Verification items for the finished model (mm, model axes). Face numbers are marked on the shaded views. A direction names the side the tool comes from. Coordinates: 2 decimals unless noted, no trailing zeros. Write each loop counter-clockwise with the first axis right and the second up, starting at its lowest first coordinate (ties: lowest second). Pieces come first, ordered by that corner, then holes.
```python
from build123d import *

# Parameters (mm, degrees)
SKETCH_1_W           = 36
SKETCH_1_H           = 20
EXTRUDE_1_DEPTH      = 8
SKETCH_2_W           = 8
SKETCH_2_H           = 20
CUT_EXTRUDE_1_DEPTH  = 3.5
SKETCH_3_R           = 2.5
CUT_EXTRUDE_2_DEPTH  = 4
SKETCH_5_W           = 7
SKETCH_5_H           = 16
CUT_EXTRUDE_4_DEPTH  = 3.5
FILLET_1_R           = 1
SKETCH_6_R           = 1.15
CUT_EXTRUDE_5_DEPTH  = 5.5
SKETCH_7_W           = 10
SKETCH_7_H           = 20
CUT_EXTRUDE_6_DEPTH  = 2
CUT_EXTRUDE_7_DEPTH  = 4
SKETCH_9_R           = 1
CUT_EXTRUDE_10_DEPTH = 3
SKETCH_10_R          = 2
CUT_EXTRUDE_11_DEPTH = 2.4
SKETCH_11_W          = 6
SKETCH_11_H          = 6
CUT_EXTRUDE_15_DEPTH = 3


with BuildPart() as part:
    # 草图1 → 凸台-拉伸1 (new body)
    with BuildSketch(Plane(origin=(0, 0, 0), x_dir=(1, 0, 0), z_dir=(0, 1, 0))):
        with Locations((-18, 10)):
            Rectangle(SKETCH_1_W, SKETCH_1_H)
    extrude(amount=EXTRUDE_1_DEPTH)

    # 草图2 → 切除-拉伸1 (cut)
    with BuildSketch(Plane(origin=(0, 8, 0), x_dir=(1, 0, 0), z_dir=(0, 1, 0))):
        with Locations((-18, 10)):
            Rectangle(SKETCH_2_W, SKETCH_2_H)
    extrude(amount=-CUT_EXTRUDE_1_DEPTH, mode=Mode.SUBTRACT)

    # 草图3 → 切除-拉伸2 (cut)
    with BuildSketch(Plane(origin=(0, 0, 0), x_dir=(-1, 0, 0), z_dir=(0, -1, 0))):
        with Locations((8, 10)):
            Circle(SKETCH_3_R)
        with Locations((28, 10)):
            Circle(SKETCH_3_R)
    extrude(amount=-CUT_EXTRUDE_2_DEPTH, mode=Mode.SUBTRACT)

    # 草图5 → 切除-拉伸4 (cut)
    with BuildSketch(Plane(origin=(0, 8, 0), x_dir=(1, 0, 0), z_dir=(0, 1, 0))):
        with Locations((-25.5, 10)):
            Rectangle(SKETCH_5_W, SKETCH_5_H)
    extrude(amount=-CUT_EXTRUDE_4_DEPTH, mode=Mode.SUBTRACT)

    # 圆角1
    fillet_1_edges = [part.edges().sort_by_distance(p)[0] for p in [
        (-29, 6.25, -2),
        (-29, 6.25, -18),
    ]]
    fillet(fillet_1_edges, radius=FILLET_1_R)

    # 草图6 → 切除-拉伸5 (cut, through all)
    with BuildSketch(Plane(origin=(0, 4.5, 0), x_dir=(1, 0, 0), z_dir=(0, 1, 0))):
        with Locations((-18, 12.5)):
            Circle(SKETCH_6_R)
        with Locations((-18, 7.5)):
            Circle(SKETCH_6_R)
    extrude(amount=-CUT_EXTRUDE_5_DEPTH, mode=Mode.SUBTRACT)

    # 草图7 → 切除-拉伸6 (cut)
    with BuildSketch(Plane(origin=(0, 8, 0), x_dir=(1, 0, 0), z_dir=(0, 1, 0))):
        with Locations((-5, 10)):
            Rectangle(SKETCH_7_W, SKETCH_7_H)
    extrude(amount=-CUT_EXTRUDE_6_DEPTH, mode=Mode.SUBTRACT)

    # 草图8 → 切除-拉伸7 (cut)
    with BuildSketch(Plane(origin=(0, 8, 0), x_dir=(1, 0, 0), z_dir=(0, 1, 0))):
        with BuildLine():
            Line((-24, 18), (-10, 18))
            ThreePointArc((-10, 18), (-9.5, 17.5), (-10, 17))
            Line((-10, 17), (-24, 17))
            ThreePointArc((-24, 17), (-24.5, 17.5), (-24, 18))
        make_face()
    extrude(amount=-CUT_EXTRUDE_7_DEPTH, mode=Mode.SUBTRACT)

    # 草图9 → 切除-拉伸10 (cut)
    with BuildSketch(Plane(origin=(0, 6, 0), x_dir=(1, 0, 0), z_dir=(0, 1, 0))):
        with Locations((-2.25, 2)):
            Circle(SKETCH_9_R)
        with Locations((-7.75, 2)):
            Circle(SKETCH_9_R)
        with Locations((-2.25, 14)):
            Circle(SKETCH_9_R)
        with Locations((-7.75, 14)):
            Circle(SKETCH_9_R)
    extrude(amount=-CUT_EXTRUDE_10_DEPTH, mode=Mode.SUBTRACT)

    # 草图10 → 切除-拉伸11 (cut)
    with BuildSketch(Plane(origin=(0, 0, 0), x_dir=(-1, 0, 0), z_dir=(0, -1, 0))):
        with Locations((18, 12.5)):
            Circle(SKETCH_10_R)
        with Locations((18, 7.5)):
            Circle(SKETCH_10_R)
    extrude(amount=-CUT_EXTRUDE_11_DEPTH, mode=Mode.SUBTRACT)

    # 草图11 → 切除-拉伸15 (cut)
    with BuildSketch(Plane(origin=(0, 0, -20), x_dir=(-1, 0, 0), z_dir=(0, 0, -1))):
        with Locations((3, 3)):
            Rectangle(SKETCH_11_W, SKETCH_11_H)
        with Locations((33, 3)):
            Rectangle(SKETCH_11_W, SKETCH_11_H)
    extrude(amount=-CUT_EXTRUDE_15_DEPTH, mode=Mode.SUBTRACT)


solid = part.part
```
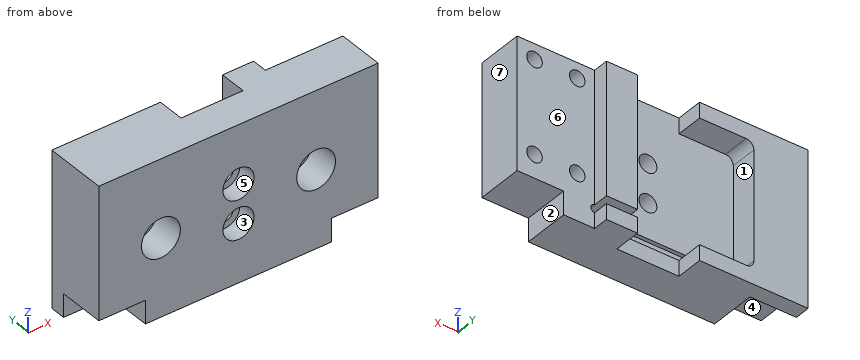
1. Material ranges on L1, parallel to X at y = 4.2, z = -2; L2, parallel to Z at x = -2.25, y = 4.3; L3, parallel to Z at x = -18, y = 3.2, recorded low to high.
2. Sectioned sample at A-A, the plane y = 1.5. Record the boundary of the cut face in (x, z).
3. Sectioned sample at D-D, the plane x = -2.25. Record the boundary of the cut face in (y, z).
4. Sectioned sample at B-B, the plane z = -10. Record the boundary of the cut face in (x, y).
5. Gauge pin test, flat ends, axial feed: P1, Ø0.6, axis at x = -17.5, z = -19, coming from the +Y side; P2, Ø3, axis at x = -33.5, y = 4, coming from the -Z side; P3, Ø2, axis at x = -18, z = -12.5, coming from the -Y side; P4, Ø1, axis at x = -28, z = -7.5, coming from the -Y side. Record the tip position at first contact, or that the pin passes through.
6. Tool access check on the marked faces 1, 2, 3 and 4. Record the directions out of +Z, -Z, +X, -X, +Y, -Y that give a thin tool (end or side, any length) a straight path to the whole face; none if there is none.
7. Sectioned sample at C-C, the plane y = 7.5. Record the boundary of the cut face in (x, z), and give its area (3 significant figures).
8. Draft check along X on the marked faces 5, 6 and 7. Enter one of: pulls with the +X half, pulls with the -X half, needs draft (parallel to the pull), parting line crosses it, or undercut.
Outcome:
1. L1: x = -36 to -8.75, -6.75 to -3.25, -1.25 to 0
1. L2: z = -17 to -15, -13 to -3, -1 to 0
1. L3: z = -20 to -13.65, -11.35 to -8.65, -6.35 to 0
2. outline: (-36, -17) - (-30, -17) - (-30, -20) - (-6, -20) - (-6, -17) - (0, -17) - (0, 0) - (-36, 0) - close; hole circle Ø5 at (-28, -10); hole circle Ø4 at (-18, -12.5); hole circle Ø4 at (-18, -7.5); hole circle Ø5 at (-8, -10)
3. outline: (0, -17) - (6, -17) - (6, -15) - (3, -15) - (3, -13) - (6, -13) - (6, -3) - (3, -3) - (3, -1) - (6, -1) - (6, 0) - (0, 0) - close
4. outline: (-36, 0) - (-30.5, 0) - (-30.5, 4) - (-25.5, 4) - (-25.5, 0) - (-10.5, 0) - (-10.5, 4) - (-5.5, 4) - (-5.5, 0) - (0, 0) - (0, 6) - (-10, 6) - (-10, 8) - (-14, 8) - (-14, 4.5) - (-29, 4.5) - (-29, 8) - (-36, 8) - close
5. P1: stops at y = 4.5
5. P2: stops at z = -17
5. P3: passes through
5. P4: stops at y = 0
6. face 1: +Y
6. face 2: -Z, +X, +Y, -Y
6. face 3: -Y
6. face 4: -Z, -X, -Y
7. outline: (-36, -20) - (-22, -20) - (-22, -18) - (-28, -18) arc R1 cw to (-29, -17) - (-29, -3) arc R1 cw to (-28, -2) - (-22, -2) - (-22, 0) - (-36, 0) - close; (-14, -20) - (-10, -20) - (-10, -18) - (-14, -18) - close; (-14, -17) - (-10, -17) - (-10, 0) - (-14, 0) - close
7. area: 244 mm2
8. face 5: undercut
8. face 6: needs draft
8. face 7: pulls with the +X half
